```python
from build123d import *

# Parameters (mm, degrees)
F0_R     = 225
F0_R_2   = 150
F1_DEPTH = 3
F2_R     = 5
F3_DEPTH = 3
F4_R     = 2.5
F5_DEPTH = 3


with BuildPart() as f1:
    # F0 (on Top) → F1 (new body)
    with BuildSketch(Plane.XY):
        Circle(F0_R)
        Circle(F0_R_2, mode=Mode.SUBTRACT)
    extrude(amount=F1_DEPTH)

    # F2 (on face) → F3 (cut)
    with BuildSketch(Plane.XY.offset(3)):
        with BuildLine():
            ThreePointArc((0, 195), (3.535534, 196.464466), (5, 200))
            ThreePointArc((5, 200), (-3.535534, 203.535534), (0, 195))
        make_face()
        with Locations((-173.205081, -100)):
            Circle(F2_R)
        with Locations((173.205081, -100)):
            Circle(F2_R)
    extrude(amount=-F3_DEPTH, mode=Mode.SUBTRACT)

    # F4 (on face) → F5 (cut)
    with BuildSketch(Plane.XY.offset(3)):
        with BuildLine():
            ThreePointArc((0, 154.5), (1.767767, 155.232233), (2.5, 157))
            ThreePointArc((2.5, 157), (-1.767767, 158.767767), (0, 154.5))
        make_face()
        with Locations((-157, 0)):
            Circle(F4_R)
        with Locations((0, -157)):
            Circle(F4_R)
        with Locations((157, 0)):
            Circle(F4_R)
    extrude(amount=-F5_DEPTH, mode=Mode.SUBTRACT)


solid = f1.part
```
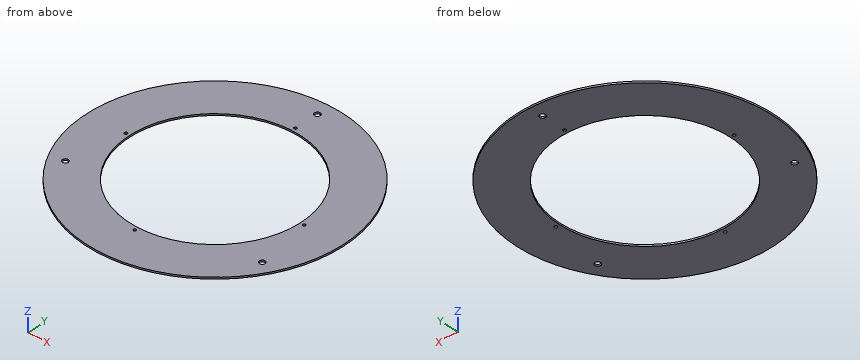
Design review of the part built by this model. Coordinates are the model's own, in mm. Coordinates: 2 decimals unless noted, no trailing zeros. Order: outer loops, then holes, each group sorted by start corner. A loop starts at its lowest first (then second) coordinate and runs counter-clockwise, first axis right, second up.
1) Take a section at C-C, the plane y = 97. Give the boundary of the cut face in (x, z).
2) Take a section at D-D, the plane x = 195. Give the boundary of the cut face in (y, z), and give its area (4 significant figures).
3) Take a section at A-A, the plane z = 2.2. State how many separate pieces and enclosed holes the cut face has, and give its area (3 significant figures).
4) Wall thickness on line 1 along Y through (x, z) = (0, 1.55); line 2 along Y through (x, z) = (-5.5, 1.2); line 3 along Y through (x, z) = (-159, 2.65): over which ranges is each line inside the solid? List them lowest first.
5) Take a section at B-B, the plane x = -20. Give the boundary of the cut face in (y, z), and give its area (3 significant figures).
6) Clearance check with a flat-ended pin moving along its axis: pin 1 (1.5 mm diameter, centred on y = 77, z = 0.5, fed in from +X). State where the tip first meets the part, or that it passes through.
Returned:
1. outline: (-203.02, 0) - (-114.42, 0) - (-114.42, 3) - (-203.02, 3) - close; (114.42, 0) - (203.02, 0) - (203.02, 3) - (114.42, 3) - close
2. outline: (-112.25, 0) - (112.25, 0) - (112.25, 3) - (-112.25, 3) - close
2. area: 673.5 mm2
3. separate pieces: 1
3. enclosed holes: 8
3. area: 88,000 mm2
4. line 1: y = -225 to -159.5, -154.5 to -150, 150 to 154.5, 159.5 to 195, 205 to 225
4. line 2: y = -224.93 to -149.9, 149.9 to 224.93
4. line 3: y = -159.2 to -1.5, 1.5 to 159.2
5. outline: (-224.11, 0) - (-148.66, 0) - (-148.66, 3) - (-224.11, 3) - close; (148.66, 0) - (224.11, 0) - (224.11, 3) - (148.66, 3) - close
5. area: 453 mm2
6. pin 1: stops at x = 211.69
